The listing builds one solid part. Answer for the finished solid, in the listing's coordinates (mm). Face numbers are marked on the shaded views. A direction names the side the tool comes from. Round coordinates to 2 decimals unless told otherwise and drop trailing zeros. Order: outer loops, then holes, each group sorted by start corner. A loop starts at its lowest first (then second) coordinate and runs counter-clockwise, first axis right, second up. Notation, with made-up numbers: M 33.25,17 L 51.25,17 A22 cw 51.25,45 Z; hole C 24,83.25 d1. An arc over 180 degrees is marked long. Write item = value, one per line. Start each with the question number.
(1) Which of the six approach directions +Z, -Z, +X, -X, +Y, -Y give full straight-line access (tool end or side, diameter ignored) to the marked faces 1 and 2?
(2) A cutting plane is placed at C-C, the plane y = -6. Determine the outline of the cut face in (x, z).
(3) Each of these flat-tipped pins is pushed along its axis until it touches: pin 1 (5 mm diameter, centred on x = -0.5, z = 87, fed in from +Y); pin 2 (0.8 mm diameter, centred on y = -17.5, z = 61, fed in from -X); pin 3 (2 mm diameter, centred on x = 18, z = 34.5, fed in from -Y). Where does it stop, or does it pass through?
(4) Straight lines are drawn through the part: probe 1 along Y at (x, z) = (0, 53); probe 2 along Y at (x, z) = (5, 89.5); probe 3 along X at (y, z) = (-7, 73). For each, find the intervals that lie inside material, in ascending order. Write a range as from..to.
(5) A cutting plane is placed at A-A, the plane x = 0. Determine the outline of the cut face in (y, z).
(6) For a pull along X with two mould halves and no side action, classify the marked faces 3 and 4 as released by +X, released by -X, zero draft, split by the parting line, or undercut.
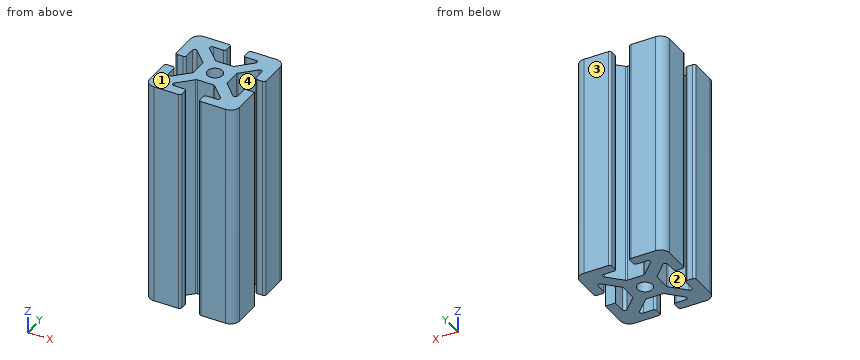
from build123d import *

# Parameters (mm, degrees)
SKIZZE1_R                       = 3.4
AUFSATZ_LINEAR_AUSTRAGEN1_DEPTH = 100
VERRUNDUNG1_R                   = 4
VERRUNDUNG2_R                   = 1


with BuildPart() as part:
    # Skizze1 → Aufsatz-Linear austragen1 (new body)
    with BuildSketch(Plane.XY):
        Polygon((-20, -20), (-4.05, -20), (-4.05, -15.5), (-11.964466094, -15.5), (-3.964466094, -7.5), (3.964466094, -7.5), (11.964466094, -15.5), (4.05, -15.5), (4.05, -20), (20, -20), (20, -4.05), (15.5, -4.05), (15.5, -11.964466094), (7.5, -3.964466094), (7.5, 3.964466094), (15.5, 11.964466094), (15.5, 4.05), (20, 4.05), (20, 20), (4.05, 20), (4.05, 15.5), (11.964466094, 15.5), (3.964466094, 7.5), (-3.964466094, 7.5), (-11.964466094, 15.5), (-4.05, 15.5), (-4.05, 20), (-20, 20), (-20, 4.05), (-15.5, 4.05), (-15.5, 11.964466094), (-7.5, 3.964466094), (-7.5, -3.964466094), (-15.5, -11.964466094), (-15.5, -4.05), (-20, -4.05), align=None)
        Circle(SKIZZE1_R, mode=Mode.SUBTRACT)
    extrude(amount=AUFSATZ_LINEAR_AUSTRAGEN1_DEPTH)

    # Verrundung1
    verrundung1_edges = [part.edges().sort_by_distance(p)[0] for p in [
        (20, -20, 50),
        (-20, -20, 50),
        (-20, 20, 50),
        (20, 20, 50),
    ]]
    fillet(verrundung1_edges, radius=VERRUNDUNG1_R)

    # Verrundung2
    verrundung2_edges = [part.edges().sort_by_distance(p)[0] for p in [
        (20, 4.05, 50),
        (15.5, 4.05, 50),
        (15.5, 11.964466094, 50),
        (7.5, 3.964466094, 50),
        (7.5, -3.964466094, 50),
        (15.5, -11.964466094, 50),
        (4.05, -20, 50),
        (4.05, -15.5, 50),
        (11.964466094, -15.5, 50),
        (3.964466094, -7.5, 50),
        (-3.964466094, -7.5, 50),
        (-11.964466094, -15.5, 50),
        (-4.05, -15.5, 50),
        (-4.05, -20, 50),
        (-20, -4.05, 50),
        (-15.5, -4.05, 50),
        (-15.5, -11.964466094, 50),
        (-7.5, -3.964466094, 50),
        (-7.5, 3.964466094, 50),
        (-15.5, 11.964466094, 50),
        (-15.5, 4.05, 50),
        (-20, 4.05, 50),
        (-4.05, 20, 50),
        (-4.05, 15.5, 50),
        (-11.964466094, 15.5, 50),
        (-3.964466094, 7.5, 50),
        (3.964466094, 7.5, 50),
        (11.964466094, 15.5, 50),
        (4.05, 15.5, 50),
        (4.05, 20, 50),
    ]]
    fillet(verrundung2_edges, radius=VERRUNDUNG2_R)


solid = part.part
Reported:
q1.face_1 = +Z, +X, -X, +Y, -Y
q1.face_2 = +Z, -Z
q2.outline = M -20,0 L -15.5,0 L -15.5,100 L -20,100 Z; M -9.54,0 L 9.54,0 L 9.54,100 L -9.54,100 Z; M 15.5,0 L 20,0 L 20,100 L 15.5,100 Z
q3.pin_1 = 7.5
q3.pin_2 = -19.85
q3.pin_3 = -19.87
q4.probe_1 = -7.5..-3.4, 3.4..7.5
q4.probe_2 = -20..-15.5, -8.54..8.54, 15.5..20
q4.probe_3 = -20..-15.5, -10.54..10.54, 15.5..20
q5.outline = M -7.5,0 L -3.4,0 L -3.4,100 L -7.5,100 Z; M 3.4,0 L 7.5,0 L 7.5,100 L 3.4,100 Z
q6.face_3 = zero draft
q6.face_4 = undercut
